Drawing for the job (mm, zero at the part's lowest x, y, z). Coordinates: 2 decimals unless noted, no trailing zeros. Order: outer loops, then holes, each group sorted by start corner. A loop starts at its lowest first (then second) coordinate and runs counter-clockwise, first axis right, second up.
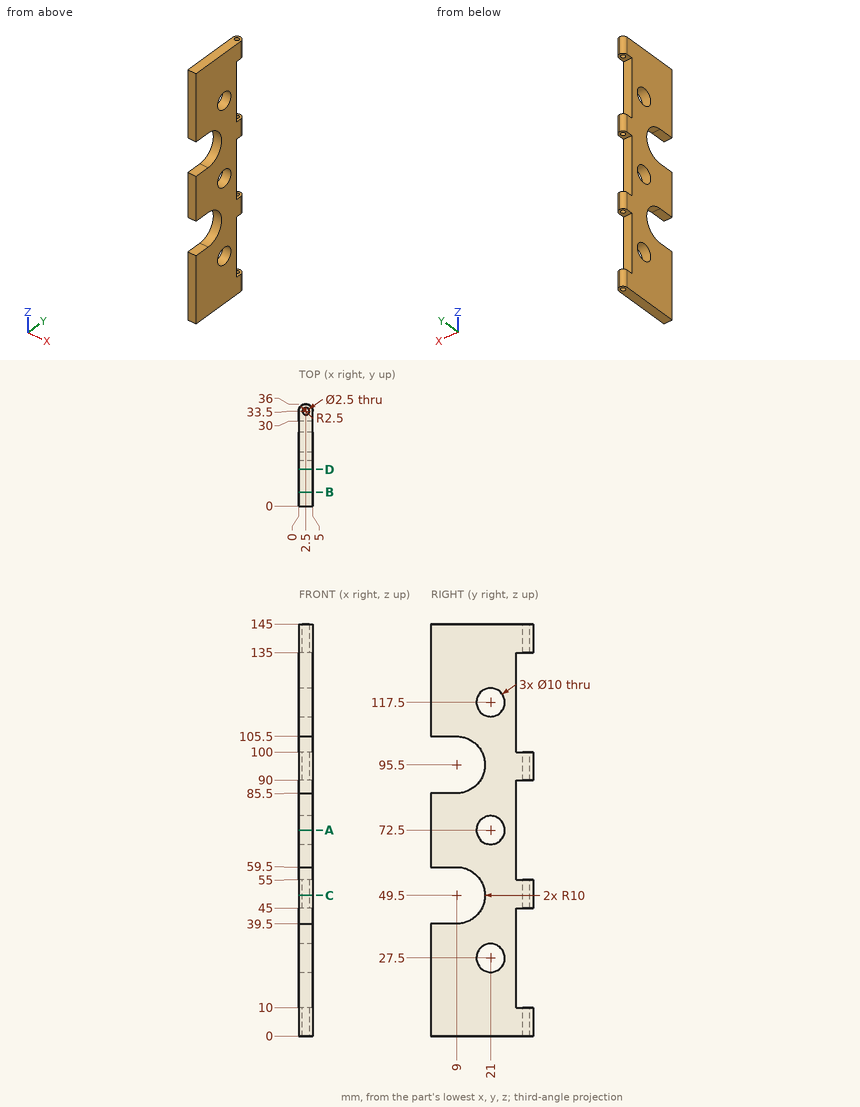
(1) Slice it at B-B, the plane y = 5. Give the cut face in (x, z).
(2) Slice it at D-D, the plane y = 13. Give the cut face in (x, z), then the cut area to 3 significant figures.
(3) Drop a flat-ended pin along its axis: pin 1 (2.5 mm diameter, centred on x = 2, z = 26.5, fed in from +Y). Give the stop position or say it passes through.
(4) Probe line 1 (Z direction, x = 3.65, y = 7); line 2 (Z direction, x = 2.4, y = 20.5); line 3 (Z direction, x = 1.65, y = 23). List the from-to ranges inside material, lowest first.
(5) Slice it at A-A, the plane z = 72.5. Give the cut face in (x, y), then the cut area to 3 significant figures.
(6) Slice it at C-C, the plane z = 49.5. Give the cut face in (x, y), then the cut area to 3 significant figures.
Here are the results:
1. outline: (0, 0) - (5, 0) - (5, 39.5) - (0, 39.5) - close; (0, 59.5) - (5, 59.5) - (5, 85.5) - (0, 85.5) - close; (0, 105.5) - (5, 105.5) - (5, 145) - (0, 145) - close
2. outline: (0, 0) - (5, 0) - (5, 40.33) - (0, 40.33) - close; (0, 58.67) - (5, 58.67) - (5, 86.33) - (0, 86.33) - close; (0, 104.67) - (5, 104.67) - (5, 145) - (0, 145) - close
2. area: 542 mm2
3. pin 1: stops at y = 30
4. line 1: z = 0 to 39.5, 59.5 to 85.5, 105.5 to 145
4. line 2: z = 0 to 22.53, 32.47 to 67.53, 77.47 to 112.53, 122.47 to 145
4. line 3: z = 0 to 22.92, 32.08 to 67.92, 77.08 to 112.92, 122.08 to 145
5. outline: (0, 0) - (5, 0) - (5, 16) - (0, 16) - close; (0, 26) - (5, 26) - (5, 30) - (0, 30) - close
5. area: 100 mm2
6. outline: (0, 19) - (5, 19) - (5, 33.5) arc R2.5 ccw to (0, 33.5) - close; hole circle Ø2.5 at (2.5, 33.5)
6. area: 77.4 mm2
